from build123d import *

# Parameters (mm, degrees)
ESQUISSE1_R        = 9
ESQUISSE1_R_2      = 6
BOSS_EXTRU_1_DEPTH = 20
ESQUISSE1_3_R      = 9
ESQUISSE1_3_R_2    = 6
BOSS_EXTRU_2_DEPTH = 60


with BuildPart() as part:
    # Esquisse1 → Boss.-Extru.1 (new body)
    # profile 1 of 2: a face of its own
    with BuildSketch(Plane.XY):
        with BuildLine():
            Line((15, 9), (0, 9))
            ThreePointArc((0, 9), (6.363961031, 6.363961031), (9, 0))
            ThreePointArc((9, 0), (6.363961031, -6.363961031), (0, -9))
            Line((0, -9), (15, -9))
            Line((15, -9), (15, 9))
        make_face()
    # profile 2 of 2: a face of its own
    with BuildSketch(Plane.XY):
        Circle(ESQUISSE1_R)
        Circle(ESQUISSE1_R_2, mode=Mode.SUBTRACT)
    extrude(amount=BOSS_EXTRU_1_DEPTH)

    # Esquisse1_3 → Boss.-Extru.2 (add)
    with BuildSketch(Plane.XY):
        with Locations(Location((0, 0, 0), (0, 0, 270))):
            Circle(ESQUISSE1_3_R)
        Circle(ESQUISSE1_3_R_2, mode=Mode.SUBTRACT)
    extrude(amount=BOSS_EXTRU_2_DEPTH)


solid = part.part
Model file for the job. Use its own axes, mm. Coordinates: 2 decimals unless noted, no trailing zeros. Loops run counter-clockwise (first coordinate to the right, second up) from the corner with the lowest first, then second, coordinate; pieces in that order, holes last. Notation, with made-up numbers: (35, 28.5) -> (72, 28.5) arc R32 ccw to (72, 57.5) -> close; hole circle Ø7 at (76.25, -25.75). An arc over 180 degrees is marked (long way). Use one line per item in the form item = value. Start each with the question number.
(1) Cut at A-A on y = 0. Give the cut face in (x, z).
(2) Flat gauge pin, fed straight in: pin 1 (1.5 mm diameter, centred on y = 5, z = 9, fed in from -X). Where does the tip first touch, or does it go through?
(3) Cut at B-B on z = 8. Give the cut face in (x, y), and give its area (3 significant figures).
(4) Cut at C-C on x = 10.25. Give the cut face in (y, z).
(5) Pull direction X, two halves, no side cores. Call faces 1 (the flat face through (8, 9, 10)), 2 (the cylindrical face through (-7.985, -4.153, 36.247)), 3 (the cylindrical face through (-6, 0, 30)): pulls with the +X half, pulls with the -X half, needs draft (parallel to the pull), parting line crosses it, or undercut.
(6) Cut at D-D on y = 8. Give the cut face in (x, z).
(7) Probe probe 1 along Y at (x, z) = (0, 18); probe 2 along Z at (x, y) = (9.5, -8); probe 3 along Y at (x, z) = (4.5, 4.5). List the from-to ranges inside material, lowest first. Write a range as from..to.
Values:
q1.outline = (-9, 0) -> (-6, 0) -> (-6, 60) -> (-9, 60) -> close; (6, 0) -> (15, 0) -> (15, 20) -> (9, 20) -> (9, 60) -> (6, 60) -> close
q2.pin_1 = -7.93
q3.outline = (0, -9) -> (15, -9) -> (15, 9) -> (0, 9) arc R9 ccw to start; hole circle Ø12 at (0, 0)
q3.area = 284 mm2
q4.outline = (-9, 0) -> (9, 0) -> (9, 20) -> (-9, 20) -> close
q5.face_1 = needs draft
q5.face_2 = parting line crosses it
q5.face_3 = undercut
q6.outline = (-4.12, 0) -> (15, 0) -> (15, 20) -> (4.12, 20) -> (4.12, 60) -> (-4.12, 60) -> close
q7.probe_1 = -9..-6, 6..9
q7.probe_2 = 0..20
q7.probe_3 = -9..-3.97, 3.97..9
